Autodesk Inventor part; units mm, degrees
ref_plane "YZ Plane" through (0, 0, 0) normal (1, 0, 0) x (0, 1, 0)
ref_plane "XZ Plane" through (0, 0, 0) normal (0, 1, 0) x (-1, 0, 0)
ref_plane "XY Plane" through (0, 0, 0) normal (0, 0, 1) x (1, 0, 0)
sketch "Sketch1" plane through (0, 0, 0) normal (0, 0, 1) x (1, 0, 0)
  line L0 (-12.7, -25.4) -> (12.7, -25.4)
  line L1 (12.7, -25.4) -> (12.7, 25.4)
  line L2 (12.7, 25.4) -> (-12.7, 25.4)
  line L3 (-12.7, 25.4) -> (-12.7, -25.4)
  line L4 (-12.7, -25.4) -> (12.7, 25.4) construction
  line L5 (12.7, -25.4) -> (-12.7, 25.4) construction
  line L6 (-9.525, 22.225) -> (9.525, 22.225)
  line L7 (9.525, 22.225) -> (9.525, -22.225)
  line L8 (9.525, -22.225) -> (-9.525, -22.225)
  line L9 (-9.525, -22.225) -> (-9.525, 22.225)
  point P0 (0, 0)
  dimension "width" = 25.4
  dimension "height" = 50.8
  dimension "thickness" = 3.175
extrude "Extrusion1" add sketch "Sketch1" along normal mid plane 127
sketch "Sketch2" plane through (12.7, -25.4, 63.5) normal (1, 0, 0) x (0, 0, -1)
  line L0 (127, 50.8) -> (0, 50.8) construction
  line L1 (0, 0) -> (0, 50.8) construction
  line L2 (127, 0) -> (0, 0) construction
  line L3 (127, 50.8) -> (127, 0) construction
  circle A0 centre (114.3, 42.8625) radius 4.7625 construction
  line L4 (0, 47.625) -> (127, 47.625) construction
  circle A1 centre (114.3, 7.9375) radius 4.7625 construction
  line L5 (0, 3.175) -> (127, 3.175) construction
  point P0 (63.5, 25.4)
  point P1 (88.9, 42.8625)
  point P2 (88.9, 7.9375)
  point P3 (63.5, 42.8625)
  point P4 (63.5, 7.9375)
  point P5 (38.1, 42.8625)
  point P6 (38.1, 7.9375)
  point P7 (12.7, 42.8625)
  point P8 (12.7, 7.9375)
  point P9 (-12.7, 42.8625)
  point P10 (-12.7, 7.9375)
  point P11 (-38.1, 42.8625)
  point P12 (-38.1, 7.9375)
  point P13 (-63.5, 42.8625)
  point P14 (-63.5, 7.9375)
  point P15 (-88.9, 42.8625)
  point P16 (-88.9, 7.9375)
  point P17 (-114.3, 42.8625)
  point P18 (-114.3, 7.9375)
  dimension "d5" = 9.525
  dimension "d6" = 9.525
  dimension "d7" = 12.7
  dimension "d10" = 25.4
hole "Hole1" at (12.7, 17.4625, -50.8) at (12.7, -17.4625, -50.8) at (12.7, 17.4625, -25.4) at (12.7, -17.4625, -25.4) at (12.7, 17.4625, 0) at (12.7, -17.4625, 0) at (12.7, 17.4625, 25.4) at (12.7, -17.4625, 25.4) at (12.7, 17.4625, 50.8) at (12.7, -17.4625, 50.8) at (12.7, 17.4625, 76.2) at (12.7, -17.4625, 76.2) at (12.7, 17.4625, 101.6) at (12.7, -17.4625, 101.6) at (12.7, 17.4625, 127) at (12.7, -17.4625, 127) at (12.7, 17.4625, 152.4) at (12.7, -17.4625, 152.4) at (12.7, 17.4625, 177.8) at (12.7, -17.4625, 177.8) direction (-1, 0, 0) diameter 5.1054 end through all
properties part number "EL2-S-001" material "Aluminum 6061"
Can you work these out from the model? Positions are in its coordinate system, mm. A direction names the side the tool comes from. Coordinates: 2 decimals unless noted, no trailing zeros. Order: outer loops, then holes, each group sorted by start corner. A loop starts at its lowest first (then second) coordinate and runs counter-clockwise, first axis right, second up. Notation, with made-up numbers: (53.25, -18.75) - (106.25, -18.75) arc R25 cw to (106.25, -1.75) - close; hole circle Ø9 at (8, 59). An arc over 180 degrees is marked (long way). Answer as a JSON object with one key per item and string values. Group by question number.
Q1. On a 3-axis mill with a long thin cutter (end or side, diameter ignored), from which of +Z, -Z, +X, -X, +Y, -Y can I reach the whole of each face in a straight line? I mean faces 5 (the face through (9.525, 0, -1)), 6 (the face through (11.09, 14.93, -50.47)). Say none if no direction works.
Q2. Imagine slicing it at C-C (y = -10). Please give me the cut outline in (x, z) (3 decimals), and give its area (3 significant figures).
Q3. We'd pull the mould along Z, two halves only. Please class faces 1 (the face through (-10, -2, 63.5)), 2 (the face through (0, -22.225, -1)), 3 (the face through (11.09, -19.615, -26.772)), 4 (the face through (11.09, -19.615, 49.428)): +Z half, -Z half, draft (parallel to the pull), parting line (faces both ways), or undercut.
Q4. Imagine slicing it at B-B (x = 6). Please give me the cut outline in (y, z) (3 decimals), and give its area (3 significant figures).
Q5. Will these pins go through, and if not, where does the flat tip stop? P1, Ø6.5, axis at y = 17.46, z = 50.8, coming from the -X side; P2, Ø3, axis at y = 17.46, z = -50.8, coming from the +X side.
Q6. Imagine slicing it at D-D (z = -50.8). Please give me the cut outline in (x, y) (3 decimals), and give its area (3 significant figures).
Q7. I need wall thicknesses on line 1 (Y direction, x = 11, z = 25.4); line 2 (X direction, y = -0.5, z = -6) (3 decimals); line 3 (Y direction, x = 7.75, z = 6) (3 decimals). Which ranges of each line are inside material? Lowest first, please. Write a range as from..to.
Q8. Imagine slicing it at A-A (z = 37.5). Please give me the cut outline in (x, y) (3 decimals), and give its area (3 significant figures).
Determined:
{
 "1": {"face 5": "+Z, -Z", "face 6": "+X, -X"},
 "2": {"outline": "(-12.7, -63.5) - (-9.525, -63.5) - (-9.525, 63.5) - (-12.7, 63.5) - close; (9.525, -63.5) - (12.7, -63.5) - (12.7, 63.5) - (9.525, 63.5) - close", "area": "806 mm2"},
 "3": {"face 1": "+Z half", "face 2": "draft", "face 3": "undercut", "face 4": "undercut"},
 "4": {"outline": "(-25.4, -63.5) - (-22.225, -63.5) - (-22.225, 63.5) - (-25.4, 63.5) - close; (22.225, -63.5) - (25.4, -63.5) - (25.4, 63.5) - (22.225, 63.5) - close", "area": "806 mm2"},
 "5": {"P1": "stops at x = -12.7", "P2": "passes through"},
 "6": {"outline": "(-12.7, -25.4) - (12.7, -25.4) - (12.7, -20.015) - (9.525, -20.015) - (9.525, -22.225) - (-9.525, -22.225) - (-9.525, -20.015) - (-12.7, -20.015) - close; (-12.7, -14.91) - (-9.525, -14.91) - (-9.525, 14.91) - (-12.7, 14.91) - close; (-12.7, 20.015) - (-9.525, 20.015) - (-9.525, 22.225) - (9.525, 22.225) - (9.525, 20.015) - (12.7, 20.015) - (12.7, 25.4) - (-12.7, 25.4) - close; (9.525, -14.91) - (12.7, -14.91) - (12.7, 14.91) - (9.525, 14.91) - close", "area": "379 mm2"},
 "7": {"line 1": "y = -25.4..-20.02, -14.91..14.91, 20.02..25.4", "line 2": "x = -12.7..-9.525, 9.525..12.7", "line 3": "y = -25.4..-22.225, 22.225..25.4"},
 "8": {"outline": "(-12.7, -25.4) - (12.7, -25.4) - (12.7, 25.4) - (-12.7, 25.4) - close; hole (-9.525, -22.225) - (9.525, -22.225) - (9.525, 22.225) - (-9.525, 22.225) - close", "area": "444 mm2"}
}
